from build123d import *

# Parameters (mm, degrees)
BOSS_EXTRUDE1_DEPTH        = 6.35
F_1_1_DIAMETER_HOLE1_D     = 28.575
F_1_1_DIAMETER_HOLE1_DEPTH = 25.4
F_1_1_DIAMETER_HOLE1_TIP   = 8.584796094


with BuildPart() as part:
    # Sketch1 → Boss-Extrude1 (new body)
    with BuildSketch(Plane.XY):
        with BuildLine():
            Line((-19.05, 0), (-19.05, 41.91))
            ThreePointArc((-19.05, 41.91), (0, 60.96), (19.05, 41.91))
            Line((19.05, 41.91), (19.05, 0))
            ThreePointArc((19.05, 0), (0, -19.05), (-19.05, 0))
        make_face()
    extrude(amount=BOSS_EXTRUDE1_DEPTH)

    # 1 (1) Diameter Hole1
    with Locations(Plane.XY.offset(6.35)):
        with Locations((0, 41.91), (0, 0)):
            Hole(F_1_1_DIAMETER_HOLE1_D / 2, depth=F_1_1_DIAMETER_HOLE1_DEPTH)
            with Locations((0, 0, -(F_1_1_DIAMETER_HOLE1_DEPTH + F_1_1_DIAMETER_HOLE1_TIP / 2))):  # 118° drill point
                Cone(0, F_1_1_DIAMETER_HOLE1_D / 2, F_1_1_DIAMETER_HOLE1_TIP, mode=Mode.SUBTRACT)


solid = part.part
Can you work these out from the model? Positions are in its coordinate system, mm. Round coordinates to 2 decimals unless told otherwise and drop trailing zeros. Write each loop counter-clockwise with the first axis right and the second up, starting at its lowest first coordinate (ties: lowest second). Pieces come first, ordered by that corner, then holes. Notation, with made-up numbers: (79.5, 7) - (129.5, 7) arc R31 cw to (129.5, 44) - close; hole circle Ø5 at (-21.75, 53). An arc over 180 degrees is marked (long way). Write each question's results on one line, items separated by ' | '. Start each with the question number.
1) For pin 1 Ø1.5 at (y, z) = (-8.5, 5.5) entering from -X; pin 2 Ø1.5 at (x, y) = (-12, -2) entering from +Z; pin 3 Ø2 at (y, z) = (43.5, 4) entering from +X, each with a flat end and sliding along its axis, tell me the tip position at first contact or that it passes through.
2) Suppose I cut it at C-C (z = 3.5). Give the number of separate pieces and of enclosed holes in the cut face, and give its area (3 significant figures).
3) We'd pull the mould along Y, two halves only. Please class faces 1 (the flat face through (19.05, 21, 3)), 2 (the cylindrical face through (0.419, -19.045, 3.131)), 3 (the cylindrical face through (3.097, 27.962, 3.131)): released by +Y, released by -Y, zero draft, split by the parting line, or undercut.
4) Suppose I cut it at B-B (y = 2). List the corners of the cut face in (x, z) for me.
5) Suppose I cut it at D-D (x = -8.5). List the corners of the cut face in (y, z) for me.
6) Please list where these lines run through material, in increasing order: line 1 (Y direction, x = 0, z = 3.5); line 2 (Y direction, x = 10, z = 3.25); line 3 (X direction, y = 41, z = 5.75).
7) Suppose I cut it at A-A (x = 0). List the corners of the cut face in (y, z) for me, and give its area (3 significant figures).
Here are the results:
1) pin 1: stops at x = -17.4 | pin 2: passes through | pin 3: stops at x = 19.04
2) separate pieces: 1 | enclosed holes: 2 | area: 1,450 mm2
3) face 1: zero draft | face 2: released by -Y | face 3: undercut
4) outline: (-19.05, 0) - (-14.15, 0) - (-14.15, 6.35) - (-19.05, 6.35) - close; (14.15, 0) - (19.05, 0) - (19.05, 6.35) - (14.15, 6.35) - close
5) outline: (-17.05, 0) - (-11.48, 0) - (-11.48, 6.35) - (-17.05, 6.35) - close; (11.48, 0) - (30.43, 0) - (30.43, 6.35) - (11.48, 6.35) - close; (53.39, 0) - (58.96, 0) - (58.96, 6.35) - (53.39, 6.35) - close
6) line 1: y = -19.05 to -14.29, 14.29 to 27.62, 56.2 to 60.96 | line 2: y = -16.21 to -10.2, 10.2 to 31.71, 52.11 to 58.12 | line 3: x = -19.05 to -14.26, 14.26 to 19.05
7) outline: (-19.05, 0) - (-14.29, 0) - (-14.29, 6.35) - (-19.05, 6.35) - close; (14.29, 0) - (27.62, 0) - (27.62, 6.35) - (14.29, 6.35) - close; (56.2, 0) - (60.96, 0) - (60.96, 6.35) - (56.2, 6.35) - close | area: 145 mm2
